from build123d import *

# Parameters (mm, degrees)
CUT_EXTRUDE_1_DEPTH      = 67.520673478
CUT_EXTRUDE_1_DEPTH_BACK = 67.520673478
SKETCH_2_R               = 2
CHAMFER_1_SIZE           = 1


with BuildPart() as part:
    # Эскиз1 → Повернуть1 (revolve)
    with BuildSketch(Plane.XY, mode=Mode.PRIVATE) as revolve_1_sk:
        Polygon((0, 0), (0, 5), (17, 5), (17, 6), (32, 6), (32, 8), (40, 8), (40, 10), (43, 10), (43, 7.5), (46.3, 7.5), (46.3, 10), (49, 10), (49, 6), (55, 6), (55, 5), (65, 5), (65, 2), (25, 2), (23.845299462, 0), align=None)
    revolve(revolve_1_sk.sketch.rotate(Axis((0, 0, 0), (1, 0, 0)), 90), axis=Axis((0, 0, 0), (1, 0, 0)))

    # Эскиз2 → Вырез-Вытянуть1 (cut, two sides: drawn at the far end of the back side and taken through both)
    with BuildSketch(Plane.XY.offset(-CUT_EXTRUDE_1_DEPTH_BACK)):
        with Locations((30, 0)):
            Circle(SKETCH_2_R)
    extrude(amount=CUT_EXTRUDE_1_DEPTH + CUT_EXTRUDE_1_DEPTH_BACK, mode=Mode.SUBTRACT)

    # Фаска1
    chamfer_1_edges = [part.edges().sort_by_distance(p)[0] for p in [
        (0, 0, -5),
    ]]
    chamfer(chamfer_1_edges, length=CHAMFER_1_SIZE)


solid = part.part
The model under review builds one solid part; all positions refer to its coordinate system, in mm. A direction names the side the tool comes from. Round coordinates to 2 decimals unless told otherwise and drop trailing zeros. Write each loop counter-clockwise with the first axis right and the second up, starting at its lowest first coordinate (ties: lowest second). Pieces come first, ordered by that corner, then holes. Notation, with made-up numbers: (56, -28.75) - (107, -28.75) arc R17 cw to (107, -10.75) - close; hole circle Ø10 at (-8, 28). An arc over 180 degrees is marked (long way). One line per item, written item: value. Start each with the question number.
1. Consider section B-B on x = 36.5. Write out the cut boundary in (y, z), and give its area (3 significant figures).
2. The part is to be moulded in two halves that separate along Y. For faces 5 (the face through (36.06, 7.81, -1.73)), 6 (the face through (65, -0.1, 2.2)), 7 (the face through (47, 0, -2)), say which applies: released by +Y, released by -Y, zero draft, split by the parting line, or undercut.
3. Clearance check with flat-ended pins moving along their axes: P1, Ø8, axis at x = 25.5, y = 7, coming from the -Z side; P2, Ø3, axis at x = 49.5, y = 2.5, coming from the -Z side; P3, Ø1.5, axis at x = 53.5, y = 5, coming from the +Z side. State where each tip first meets the part, or that it passes through.
4. To check wall thickness, follow L1, parallel to Y at x = 28.05, z = 0; L2, parallel to X at y = -8, z = -1; L3, parallel to Y at x = 61, z = -3. State the ranges of each line that lie inside material, in increasing order. Write a range as from..to.
5. Consider section A-A on y = 8.75. Write out the cut boundary in (x, z).
6. Machinability: for faces 1 (the face through (9, 0, -5)), 2 (the face through (55, -4, -4)), 3 (the face through (46.3, -7, -4)), 4 (the face through (28, 0, 4)), which of the approach directions +Z, -Z, +X, -X, +Y, -Y give a long, thin tool a straight path to every point of the face, cutting with its end or side? Answer none if there is none.
7. Consider section C-C on x = 19.5. Write out the cut boundary in (y, z), and give its area (3 significant figures).
Checks:
1. outline: circle Ø16 at (0, 0); hole circle Ø4 at (0, 0)
1. area: 188 mm^2
2. face 5: split by the parting line
2. face 6: zero draft
2. face 7: undercut
3. P1: stops at z = -5.2
3. P2: stops at z = -9.94
3. P3: stops at z = 4.24
4. L1: y = -6..-2, 2..6
4. L2: x = 40..43, 46.3..49
4. L3: y = -4..4
5. outline: (40, -4.84) - (43, -4.84) - (43, 4.84) - (40, 4.84) - close; (46.3, -4.84) - (49, -4.84) - (49, 4.84) - (46.3, 4.84) - close
6. face 1: -X
6. face 2: +X
6. face 3: none
6. face 4: +Z, -Z
7. outline: circle Ø12 at (0, 0)
7. area: 113 mm^2
